Autodesk Inventor part; units mm, degrees
ref_plane "YZ Plane" through (0, 0, 0) normal (1, 0, 0) x (0, 1, 0)
ref_plane "XZ Plane" through (0, 0, 0) normal (0, 1, 0) x (-1, 0, 0)
ref_plane "XY Plane" through (0, 0, 0) normal (0, 0, 1) x (1, 0, 0)
sketch "Sketch1" plane through (0, 0, 0) normal (0, 1, 0) x (-1, 0, 0)
  line L0 (0, 17.637) -> (-76.2, 17.637)
  line L1 (-76.2, 17.637) -> (-76.2, -17.863)
  line L2 (-76.2, -17.863) -> (0, -17.863)
  line L3 (0, -17.863) -> (0, 17.637)
  line L4 (0, 17.637) -> (15.748, 17.637)
  line L5 (15.748, 17.637) -> (15.748, -17.863)
  line L6 (15.748, -17.863) -> (0, -17.863)
  line L7 (0, -17.863) -> (0, 17.637)
  circle A0 centre (-44.068, -12.113) radius 1.7
  circle A1 centre (-68.068, -12.113) radius 1.7
  circle A2 centre (-44.068, 11.887) radius 1.7
  circle A3 centre (-68.068, 11.887) radius 1.7
  point P0 (0, 0)
  dimension "d0" = 76.2
  dimension "d1" = 35.5
  dimension "d2" = 17.637
  dimension "d3" = 15.748
  dimension "d45" = 3.4
  dimension "d47" = 5.75
  dimension "d50" = 24
  dimension "d53" = 24
  dimension "d58" = 44.068
extrude "Extrusion1" add sketch "Sketch1" along normal blind 4
sketch "Sketch4" plane through (0, 0, 0) normal (0, -1, 0) x (1, 0, 0)
  line L0 (-12.7, 3.175) -> (12.7, 3.175) construction
  line L1 (12.7, 3.175) -> (12.7, -3.175) construction
  line L2 (12.7, -3.175) -> (-12.7, -3.175) construction
  line L3 (-12.7, -3.175) -> (-12.7, 3.175) construction
  line L4 (-6.35, 3.175) -> (-6.35, -3.175) construction
  line L5 (6.35, 3.175) -> (6.35, -3.175) construction
  line L6 (-6.35, 3.683) -> (-13.208, 3.683)
  line L7 (-13.208, 3.683) -> (-13.208, 6.223)
  line L8 (-13.208, 6.223) -> (-6.35, 6.223)
  line L9 (-6.35, 6.223) -> (-6.35, 3.683)
  line L10 (-13.208, 6.223) -> (-15.748, 6.223)
  line L11 (-15.748, 6.223) -> (-15.748, 0)
  line L12 (-15.748, 0) -> (-13.208, 0)
  line L13 (-13.208, 0) -> (-13.208, 6.223)
  line L14 (-12.7, 0) -> (12.7, 0) construction
  line L15 (0, 3.175) -> (0, -3.175) construction
  line L16 (-6.35, -3.683) -> (-13.208, -3.683)
  line L17 (-13.208, -6.223) -> (-6.35, -6.223)
  line L18 (-6.35, -6.223) -> (-6.35, -3.683)
  line L19 (-13.208, -6.223) -> (-15.748, -6.223)
  line L20 (-15.748, -6.223) -> (-15.748, 0)
  line L21 (-13.208, 0) -> (-13.208, -6.223)
  line L22 (6.35, 3.683) -> (13.208, 3.683)
  line L23 (13.208, 3.683) -> (13.208, 6.223)
  line L24 (13.208, 6.223) -> (6.35, 6.223)
  line L25 (6.35, 6.223) -> (6.35, 3.683)
  line L26 (13.208, 6.223) -> (15.748, 6.223)
  line L27 (15.748, 6.223) -> (15.748, 0)
  line L28 (15.748, 0) -> (13.208, 0)
  line L29 (13.208, 0) -> (13.208, 6.223)
  line L30 (6.35, -6.223) -> (6.35, -3.683)
  line L31 (6.35, -3.683) -> (13.208, -3.683)
  line L32 (13.208, -6.223) -> (6.35, -6.223)
  line L33 (13.208, 0) -> (13.208, -6.223)
  line L34 (15.748, -6.223) -> (15.748, 0)
  line L35 (13.208, -6.223) -> (15.748, -6.223)
  point P0 (0, 0)
  dimension "d20" = 25.4
  dimension "d21" = 6.35
  dimension "d22" = 3.175
  dimension "d23" = 12.7
  dimension "d24" = 6.35
  dimension "d25" = 6.35
  dimension "d26" = 6.858
  dimension "d27" = 2.54
  dimension "d28" = 0.508
  dimension "d29" = 2.54
  dimension "d30" = 6.223
extrude "Extrusion5" add sketch "Sketch4" along normal blind 6.35
sketch "Sketch6" plane through (0, 0, 0) normal (0, -1, 0) x (1, 0, 0)
  circle A0 centre (27.432, 0) radius 9.525
  line L0 (0, 24.737) -> (0, -24.963)
  point P0 (0, 0)
  dimension "d35" = 19.05
  dimension "d36" = 27.432
extrude "Extrusion7" add sketch "Sketch6" along normal blind 3
sketch "Sketch7" plane through (27.432, -3, 0) normal (0, -1, 0) x (1, 0, 0)
  circle A0 centre (0, 0) radius 1.7
  point P0 (-27.432, 0)
  dimension "d39" = 3.4
extrude "Extrusion8" cut sketch "Sketch7" against normal through all
sketch "Sketch8" plane through (0, 0, 0) normal (0, -1, 0) x (1, 0, 0)
  circle A0 centre (27.432, 0) radius 1.7 construction
  line L0 (27.432, 0) -> (15.875, -6.35) construction
  line L1 (27.432, 0) -> (15.875, 0) construction
  line L2 (6.35, -6.223) -> (6.35, -3.683) construction
  line L3 (27.432, 0) -> (6.35, -6.223) construction
  line L4 (27.432, 0) -> (6.35, 3.6065) construction
  point P0 (0, 0)
sketch "Sketch9" plane through (0, 4, 0) normal (0, 1, 0) x (1, 0, 0)
  circle A0 centre (27.432, 0) radius 1.7 construction
  circle A1 centre (27.432, 0) radius 3.25 construction
  line L0 (27.432, 3.25) -> (30.2466, 1.625)
  line L1 (30.2466, 1.625) -> (30.2466, -1.625)
  line L2 (30.2466, -1.625) -> (27.432, -3.25)
  line L3 (27.432, -3.25) -> (24.6174, -1.625)
  line L4 (24.6174, -1.625) -> (24.6174, 1.625)
  line L5 (24.6174, 1.625) -> (27.432, 3.25)
  point P0 (0, 0)
  dimension "d42" = 6.5
extrude "Extrusion9" cut sketch "Sketch9" against normal blind 2.5
sketch "Sketch10" plane through (0, 0, 0) normal (0, -1, 0) x (1, 0, 0)
  line L0 (-13.208, 3.683) -> (-13.208, -3.683)
  line L1 (13.208, 3.683) -> (6.35, 3.683)
  line L2 (-13.208, -3.683) -> (13.208, -3.683)
  line L3 (13.208, -3.683) -> (13.208, 3.683)
  line L4 (13.208, 3.683) -> (-13.208, 3.683)
  line L5 (-13.208, 3.683) -> (-13.208, -3.683)
  point P0 (0, 0)
extrude "Extrusion10" add sketch "Sketch10" along normal blind 0.5
properties part number "capstone hook mount"
Check sheet for the modelled part. Datum: model origin and axes. Units: mm. A direction names the side the tool comes from. Give positions to 0.01 mm unless a question says otherwise; leave off trailing zeros. Write each loop counter-clockwise with the first axis right and the second up, starting at its lowest first coordinate (ties: lowest second). Pieces come first, ordered by that corner, then holes. Notation, with made-up numbers: (-30.75, -3) -> (8.25, -3) arc R12 cw to (8.25, 13) -> close; hole circle Ø2 at (-21.75, 61.25). An arc over 180 degrees is marked (long way). Use one line per item in the form item = value. Start each with the question number.
1. Thickness scan on line 1 along X through (y, z) = (-4.5, -5.5); line 2 along X through (y, z) = (2.5, 10.5); line 3 along X through (y, z) = (-2.5, -4). Record the ranges inside material, lowest first. Write a range as from..to.
2. Section check C-C (z = 0). Record the cut outline in (x, y), and give its area (3 significant figures).
3. Section check B-B (x = 11). Record the cut outline in (y, z), and give its area (3 significant figures).
4. Section check A-A (y = -1.5). Record the cut outline in (x, z) (3 decimals).
5. Section check D-D (y = -5.5). Record the cut outline in (x, z), and give its area (3 significant figures).
6. Go/stop test with flat-tipped pins: P1, Ø3, axis at x = -12, y = -3.5, coming from the +Z side; P2, Ø1.8, axis at x = -10.5, y = -2.5, coming from the -Z side; P3, Ø21, axis at x = 24, z = 1, coming from the -Y side; P4, Ø3, axis at x = 7.5, z = -8.5, coming from the -Y side. Record where each tip stops, or that it passes through.
7. Mould release check, pull along X, two halves, no side actions. Record for faces 1 (the flat face through (76.2, 2, 0)), 2 (the flat face through (-10, -3, -3.683)), 3 (the flat face through (-11, -3, 6.223)): pulls with the +X half, pulls with the -X half, needs draft (parallel to the pull), parting line crosses it, or undercut.
8. Access from +Z, -Z, +X, -X, +Y, -Y to the whole of each face (thin tool, end or side, straight path). Record for faces 4 (the flat face through (26.005, 2.768, -2.426)), 5 (the flat face through (15.748, -3, 0)), 6 (the flat face through (11, -3, -6.223)).
Conclusion:
q1.line_1 = -15.75..-6.35, 6.35..15.75
q1.line_2 = -15.75..43.09, 45.05..67.09, 69.05..76.2
q1.line_3 = -15.75..-6.35, 6.35..15.75, 18.79..36.08
q2.outline = (-15.75, -6.35) -> (-13.21, -6.35) -> (-13.21, -0.5) -> (13.21, -0.5) -> (13.21, -6.35) -> (15.75, -6.35) -> (15.75, 0) -> (17.91, 0) -> (17.91, -3) -> (25.73, -3) -> (25.73, 1.5) -> (24.62, 1.5) -> (24.62, 4) -> (-15.75, 4) -> close; (29.13, -3) -> (36.96, -3) -> (36.96, 0) -> (76.2, 0) -> (76.2, 4) -> (30.25, 4) -> (30.25, 1.5) -> (29.13, 1.5) -> close
q2.area = 441 mm²
q3.outline = (-6.35, -6.22) -> (0, -6.22) -> (0, -17.86) -> (4, -17.86) -> (4, 17.64) -> (0, 17.64) -> (0, 6.22) -> (-6.35, 6.22) -> (-6.35, 3.68) -> (-0.5, 3.68) -> (-0.5, -3.68) -> (-6.35, -3.68) -> close
q3.area = 178 mm²
q4.outline = (-15.748, -6.223) -> (-6.35, -6.223) -> (-6.35, -3.683) -> (-13.208, -3.683) -> (-13.208, 3.683) -> (-6.35, 3.683) -> (-6.35, 6.223) -> (-15.748, 6.223) -> close; (6.35, -6.223) -> (15.748, -6.223) -> (15.748, 6.223) -> (6.35, 6.223) -> (6.35, 3.683) -> (13.208, 3.683) -> (13.208, -3.683) -> (6.35, -3.683) -> close; circle Ø19.05 at (27.432, 0); hole circle Ø3.4 at (27.432, 0)
q5.outline = (-15.75, -6.22) -> (-6.35, -6.22) -> (-6.35, -3.68) -> (-13.21, -3.68) -> (-13.21, 3.68) -> (-6.35, 3.68) -> (-6.35, 6.22) -> (-15.75, 6.22) -> close; (6.35, -6.22) -> (15.75, -6.22) -> (15.75, 6.22) -> (6.35, 6.22) -> (6.35, 3.68) -> (13.21, 3.68) -> (13.21, -3.68) -> (6.35, -3.68) -> close
q5.area = 133 mm²
q6.P1 = 6.22
q6.P2 = -6.22
q6.P3 = -6.35
q6.P4 = 0
q7.face_1 = pulls with the +X half
q7.face_2 = undercut
q7.face_3 = needs draft
q8.face_4 = +Y
q8.face_5 = +Z, -Z, -Y
q8.face_6 = -Z, -X, -Y
